from build123d import *

# Parameters (mm, degrees)
BOSS_EXTRUDE2_DEPTH         = 12.7
SKETCH3_W                   = 25.4
SKETCH3_H                   = 25.4
CUT_EXTRUDE1_DEPTH          = 26.4
CUT_EXTRUDE3_DEPTH          = 26.4
HOLE1_D                     = 6.477
HOLE1_DEPTH                 = 14.2748
F_3_8_16_TAPPED_HOLE1_D     = 7.9375
F_3_8_16_TAPPED_HOLE1_DEPTH = 20.32
F_3_8_16_TAPPED_HOLE1_TIP   = 2.384665582
CHAMFER1_SIZE               = 1.524


with BuildPart() as part:
    # Sketch2 → Boss-Extrude2 (new body, symmetric)
    with BuildSketch(Plane(origin=(0, 0, 0), x_dir=(1, 0, 0), z_dir=(0, 1, 0))):
        Polygon((0, 36.5125), (0, -36.5125), (63.5, -36.5125), (88.9, -18.9865), (88.9, 18.9865), (63.5, 36.5125), align=None)
    extrude(amount=BOSS_EXTRUDE2_DEPTH, both=True)

    # Sketch3 → Cut-Extrude1 (cut, through all)
    with BuildSketch(Plane(origin=(0, 12.7, 0), x_dir=(1, 0, 0), z_dir=(0, 1, 0))):
        with Locations((76.2, 0)):
            Rectangle(SKETCH3_W, SKETCH3_H)
    extrude(amount=-CUT_EXTRUDE1_DEPTH, mode=Mode.SUBTRACT)

    # Sketch4 → Cut-Extrude3 (cut, through all)
    with BuildSketch(Plane(origin=(0, 12.7, 0), x_dir=(1, 0, 0), z_dir=(0, 1, 0))):
        with BuildLine():
            Line((0, 7.9375), (12.6873, 7.9375))
            ThreePointArc((12.6873, 7.9375), (20.6248, 0), (12.6873, -7.9375))
            Line((12.6873, -7.9375), (0, -7.9375))
            Line((0, -7.9375), (0, 7.9375))
        make_face()
    extrude(amount=-CUT_EXTRUDE3_DEPTH, mode=Mode.SUBTRACT)

    # Hole1
    with Locations(Plane(origin=(0, 12.7, 0), x_dir=(1, 0, 0), z_dir=(0, 1, 0))):
        with Locations((26.9748, 0)):
            Hole(HOLE1_D / 2, depth=HOLE1_DEPTH)

    # 3/8-16 Tapped Hole1
    with Locations(Plane(origin=(63.5, 0, 0), x_dir=(0, 0, -1), z_dir=(1, 0, 0))):
        with Locations((0, 0)):
            Hole(F_3_8_16_TAPPED_HOLE1_D / 2, depth=F_3_8_16_TAPPED_HOLE1_DEPTH)
            with Locations((0, 0, -(F_3_8_16_TAPPED_HOLE1_DEPTH + F_3_8_16_TAPPED_HOLE1_TIP / 2))):  # 118° drill point
                Cone(0, F_3_8_16_TAPPED_HOLE1_D / 2, F_3_8_16_TAPPED_HOLE1_TIP, mode=Mode.SUBTRACT)

    # Chamfer1
    chamfer1_edges = [part.edges().sort_by_distance(p)[0] for p in [
        (31.75, 12.7, 36.5125),
        (76.2, 12.7, 27.7495),
        (88.9, 12.7, 15.84325),
        (76.2, 12.7, -27.7495),
        (88.9, 12.7, -15.84325),
        (0, 12.7, 22.225),
        (31.75, 12.7, -36.5125),
        (0, 12.7, -22.225),
    ]]
    chamfer(chamfer1_edges, length=CHAMFER1_SIZE)


solid = part.part
Can you work these out from the model? Positions are in its coordinate system, mm. A direction names the side the tool comes from. Give positions to 0.01 mm unless a question says otherwise; leave off trailing zeros. Order: outer loops, then holes, each group sorted by start corner. A loop starts at its lowest first (then second) coordinate and runs counter-clockwise, first axis right, second up. Notation, with made-up numbers: M 17.25,-21 L 57.25,-21 A20 cw 57.25,16 Z; hole C 29,79 d10. An arc over 180 degrees is marked long. One line per item, written item: value.
Item 1: If we section it at D-D on z = -22.5: Write out the boundary of the cut face in (x, y).
Verdict:
outline: M 0,-12.7 L 83.81,-12.7 L 83.81,11.18 L 81.12,12.7 L 1.52,12.7 L 0,11.18 Z
Item 2: If we section it at B-B on y = -5.25: Write out the boundary of the cut face in (x, z) (1 decimal).
Verdict:
outline: M 0,-36.5 L 63.5,-36.5 L 88.9,-19 L 88.9,-12.7 L 63.5,-12.7 L 63.5,12.7 L 88.9,12.7 L 88.9,19 L 63.5,36.5 L 0,36.5 L 0,7.9 L 12.7,7.9 A7.9 cw 12.7,-7.9 L 0,-7.9 Z
Item 3: For faces 5 (the face through (76, 0, -12.7)), 6 (the face through (53.198, -3.874, -0.86)), 7 (the face through (76.378, -0.595, -27.627)), which set-ups out of +Z, -Z, +X, -X, +Y, -Y let a thin tool reach every point of the face, with its end or its side?
Verdict:
face 5: +X, +Y, -Y
face 6: +X
face 7: -Z, +X, +Y, -Y
Item 4: For pin 1 (5 mm diameter, centred on x = 17.5, z = 6, fed in from +Y); pin 2 (12.5 mm diameter, centred on x = 82, y = 0, fed in from +Z); pin 3 (1 mm diameter, centred on y = 5.5, z = -5, fed in from -X); pin 4 (4 mm diameter, centred on x = 26.97, z = 0, fed in from +Y), each with a flat end and sliding along its axis, tell me the tip position at first contact or that it passes through.
Verdict:
pin 1: y = 12.7
pin 2: z = 28.06
pin 3: x = 18.41
pin 4: y = -1.57
Item 5: If we mould it in two halves opening along X, with no side actions, what happens to faces 1 (the face through (27, -1.575, 0)), 2 (the face through (23.983, 5.463, 1.24)), 3 (the face through (88.9, -1, -16)), 4 (the face through (6, 0, 7.938))? For each: pulls with the +X half, pulls with the -X half, needs draft (parallel to the pull), parting line crosses it, or undercut.
Verdict:
face 1: undercut
face 2: undercut
face 3: pulls with the +X half
face 4: needs draft
Item 6: Please list where these lines run through material, in increasing order: line 1 (Z direction, x = 58.5, y = 0); line 2 (Z direction, x = 10.5, y = 1.75); line 3 (Y direction, x = 56, z = 0).
Verdict:
line 1: -36.51 to -3.97, 3.97 to 36.51
line 2: -36.51 to -7.94, 7.94 to 36.51
line 3: -12.7 to -3.97, 3.97 to 12.7
Item 7: If we section it at C-C on x = 14: Write out the boundary of the cut face in (y, z).
Verdict:
outline: M -12.7,-36.51 L 11.18,-36.51 L 12.7,-34.99 L 12.7,-7.83 L -12.7,-7.83 Z; M -12.7,7.83 L 12.7,7.83 L 12.7,34.99 L 11.18,36.51 L -12.7,36.51 Z
Item 8: If we section it at A-A on y = 9.5: Write out the boundary of the cut face in (x, z) (1 decimal), and give its area (3 significant figures).
Verdict:
outline: M 0,-36.5 L 63.5,-36.5 L 88.9,-19 L 88.9,-12.7 L 63.5,-12.7 L 63.5,12.7 L 88.9,12.7 L 88.9,19 L 63.5,36.5 L 0,36.5 L 0,7.9 L 12.7,7.9 A7.9 cw 12.7,-7.9 L 0,-7.9 Z; hole C 27,0 d6.5
area: 5,070 mm2
